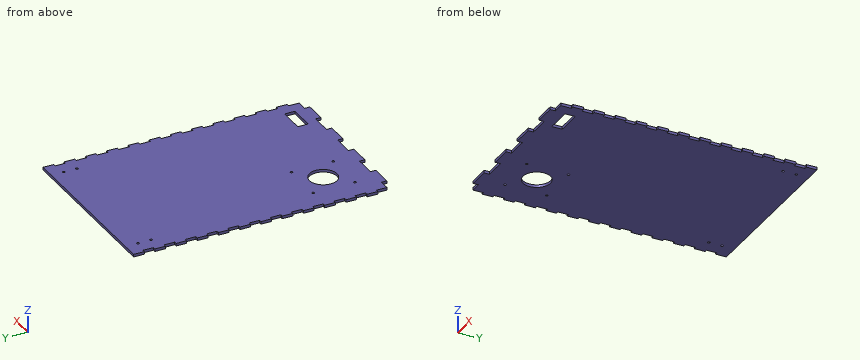
```python
from build123d import *

# Parameters (mm, degrees)
SKETCH1_W           = 203.2
SKETCH1_H           = 304.8
BOSS_EXTRUDE1_DEPTH = 3.175
SKETCH2_W           = 3.175
SKETCH2_H           = 12.7
SKETCH2_W_2         = 25.4
SKETCH2_H_2         = 6.35
BOSS_EXTRUDE2_DEPTH = 3.175
SKETCH4_R           = 16.5
SKETCH4_R_2         = 1.5
CUT_EXTRUDE1_DEPTH  = 3.175
SKETCH5_R           = 1.5
CUT_EXTRUDE2_DEPTH  = 3.175
SKETCH7_W           = 30.575
SKETCH7_H           = 12.439028
CUT_EXTRUDE4_DEPTH  = 3.175


with BuildPart() as part:
    # Sketch1 → Boss-Extrude1 (new body)
    with BuildSketch(Plane.XY):
        with Locations((101.6, 152.4)):
            Rectangle(SKETCH1_W, SKETCH1_H)
    extrude(amount=BOSS_EXTRUDE1_DEPTH)

    # Sketch2 → Boss-Extrude2 (add)
    with BuildSketch(Plane.XY.offset(3.175)):
        with Locations((-1.5875, 298.45)):
            Rectangle(SKETCH2_W, SKETCH2_H)
        with Locations((204.7875, 298.45)):
            Rectangle(SKETCH2_W, SKETCH2_H)
        with Locations((-1.5875, 273.05)):
            Rectangle(SKETCH2_W, SKETCH2_H)
        with Locations((204.7875, 273.05)):
            Rectangle(SKETCH2_W, SKETCH2_H)
        with Locations((-1.5875, 247.65)):
            Rectangle(SKETCH2_W, SKETCH2_H)
        with Locations((204.7875, 247.65)):
            Rectangle(SKETCH2_W, SKETCH2_H)
        with Locations((-1.5875, 222.25)):
            Rectangle(SKETCH2_W, SKETCH2_H)
        with Locations((204.7875, 222.25)):
            Rectangle(SKETCH2_W, SKETCH2_H)
        with Locations((-1.5875, 196.85)):
            Rectangle(SKETCH2_W, SKETCH2_H)
        with Locations((204.7875, 196.85)):
            Rectangle(SKETCH2_W, SKETCH2_H)
        with Locations((-1.5875, 171.45)):
            Rectangle(SKETCH2_W, SKETCH2_H)
        with Locations((204.7875, 171.45)):
            Rectangle(SKETCH2_W, SKETCH2_H)
        with Locations((-1.5875, 146.05)):
            Rectangle(SKETCH2_W, SKETCH2_H)
        with Locations((204.7875, 146.05)):
            Rectangle(SKETCH2_W, SKETCH2_H)
        with Locations((-1.5875, 120.65)):
            Rectangle(SKETCH2_W, SKETCH2_H)
        with Locations((204.7875, 120.65)):
            Rectangle(SKETCH2_W, SKETCH2_H)
        with Locations((-1.5875, 95.25)):
            Rectangle(SKETCH2_W, SKETCH2_H)
        with Locations((204.7875, 95.25)):
            Rectangle(SKETCH2_W, SKETCH2_H)
        with Locations((-1.5875, 69.85)):
            Rectangle(SKETCH2_W, SKETCH2_H)
        with Locations((204.7875, 69.85)):
            Rectangle(SKETCH2_W, SKETCH2_H)
        with Locations((-1.5875, 44.45)):
            Rectangle(SKETCH2_W, SKETCH2_H)
        with Locations((204.7875, 44.45)):
            Rectangle(SKETCH2_W, SKETCH2_H)
        with Locations((-1.5875, 19.05)):
            Rectangle(SKETCH2_W, SKETCH2_H)
        with Locations((204.7875, 19.05)):
            Rectangle(SKETCH2_W, SKETCH2_H)
        with Locations((25.4, -3.175)):
            Rectangle(SKETCH2_W_2, SKETCH2_H_2)
        with Locations((76.2, -3.175)):
            Rectangle(SKETCH2_W_2, SKETCH2_H_2)
        with Locations((127, -3.175)):
            Rectangle(SKETCH2_W_2, SKETCH2_H_2)
        with Locations((177.8, -3.175)):
            Rectangle(SKETCH2_W_2, SKETCH2_H_2)
    extrude(amount=-BOSS_EXTRUDE2_DEPTH)

    # Sketch4 → Cut-Extrude1 (cut)
    with BuildSketch(Plane.XY.offset(3.175)):
        with Locations((50.8, 50)):
            Circle(SKETCH4_R)
        with Locations((25.8, 75)):
            Circle(SKETCH4_R_2)
        with Locations((75.8, 75)):
            Circle(SKETCH4_R_2)
        with Locations((75.8, 25)):
            Circle(SKETCH4_R_2)
        with Locations((25.8, 25)):
            Circle(SKETCH4_R_2)
    extrude(amount=-CUT_EXTRUDE1_DEPTH, mode=Mode.SUBTRACT)

    # Sketch5 → Cut-Extrude2 (cut)
    with BuildSketch(Plane(origin=(0, 0, 0), x_dir=(-1, 0, 0), z_dir=(0, 0, -1))):
        with Locations((-187.325, 289.8)):
            Circle(SKETCH5_R)
        with Locations((-187.325, 274.05)):
            Circle(SKETCH5_R)
        with Locations(Location((-15.875, 274.05, 0), (0, 0, 180))):
            Circle(SKETCH5_R)
        with Locations(Location((-15.875, 289.8, 0), (0, 0, 180))):
            Circle(SKETCH5_R)
    extrude(amount=-CUT_EXTRUDE2_DEPTH, mode=Mode.SUBTRACT)

    # Sketch7 → Cut-Extrude4 (cut)
    with BuildSketch(Plane.XY.offset(3.175)):
        with Locations((174.3, 18.230486)):
            Rectangle(SKETCH7_W, SKETCH7_H)
    extrude(amount=-CUT_EXTRUDE4_DEPTH, mode=Mode.SUBTRACT)


solid = part.part
```
Verification items for the finished model (mm, model axes). Give positions to 0.01 mm unless a question says otherwise; leave off trailing zeros. Order: outer loops, then holes, each group sorted by start corner. A loop starts at its lowest first (then second) coordinate and runs counter-clockwise, first axis right, second up. Notation, with made-up numbers: M 77.25,70.5 L 93.25,70.5 A19 cw 93.25,89.5 Z; hole C 70.5,43 d10. An arc over 180 degrees is marked long. Answer in a Markdown table with one row per item. Add a question column.
Item 1: Section check B-B, the plane z = 1.4. State how many separate pieces and enclosed holes the cut face has, and give its area (3 significant figures).
Item 2: Section check C-C, the plane y = 235.5. Enter the section's corners in (x, z) (3 decimals), and give its area (3 significant figures).
Item 3: Scan lines: probe 1 along X at (y, z) = (75, 1.05) (3 decimals); probe 2 along Y at (x, z) = (25.8, 2.2); probe 3 along X at (y, z) = (289.8, 0.7) (3 decimals). Record each from-to range of solid material in increasing order. Write a range as from..to.
Item 4: Section check A-A, the plane x = 50.8. Enter the section's corners in (y, z) (3 decimals), and give its area (3 significant figures).
Item 5: Section check D-D, the plane x = 149. Enter the section's corners in (y, z) (3 decimals).
Item 6: Gauge pin test, flat end, axial feed: pin 1 (1 mm diameter, centred on y = 156, z = 2, fed in from +X). Record the tip position at first contact, or that the pin passes through.
Filled sheet:
| question | item | result |
|---|---|---|
| 1 | separate pieces | 1 |
| 1 | enclosed holes | 10 |
| 1 | area | 62,300 mm^2 |
| 2 | outline | M 0,0 L 203.2,0 L 203.2,3.175 L 0,3.175 Z |
| 2 | area | 645 mm^2 |
| 3 | probe 1 | x = -3.175..24.3, 27.3..74.3, 77.3..206.375 |
| 3 | probe 2 | y = -6.35..23.5, 26.5..73.5, 76.5..304.8 |
| 3 | probe 3 | x = 0..14.375, 17.375..185.825, 188.825..203.2 |
| 4 | outline | M 0,0 L 33.5,0 L 33.5,3.175 L 0,3.175 Z; M 66.5,0 L 304.8,0 L 304.8,3.175 L 66.5,3.175 Z |
| 4 | area | 863 mm^2 |
| 5 | outline | M 0,0 L 304.8,0 L 304.8,3.175 L 0,3.175 Z |
| 6 | pin 1 | stops at x = 203.2 |
